Check sheet for the modelled part. Datum: model origin and axes. Units: mm. Coordinates: 2 decimals unless noted, no trailing zeros. Write each loop counter-clockwise with the first axis right and the second up, starting at its lowest first coordinate (ties: lowest second). Pieces come first, ordered by that corner, then holes. Notation, with made-up numbers: M 75.5,-32.5 L 79.5,-32.5 A24 cw 79.5,-0.5 Z; hole C 59,2 d9. An arc over 180 degrees is marked long. Answer as CSV lines item,"result".
from build123d import *
from build123d.topology import SkipClean

# Parameters (mm, degrees)
SKETCH1_R           = 39.35
BOSS_EXTRUDE1_DEPTH = 5
SKETCH2_R           = 34.4
CUT_EXTRUDE1_DEPTH  = 5
CUT_EXTRUDE2_START  = -5
CUT_EXTRUDE2_DEPTH  = 5
BOSS_EXTRUDE2_START = -5
BOSS_EXTRUDE2_DEPTH = 5
BOSS_EXTRUDE3_START = -5
BOSS_EXTRUDE3_DEPTH = 5
SKETCH11_R          = 1.5
CUT_EXTRUDE3_DEPTH  = 5
SKETCH12_R          = 1.5
CUT_EXTRUDE4_DEPTH  = 5


with BuildPart() as part:
    # Sketch1 → Boss-Extrude1 (new body)
    with BuildSketch(Plane(origin=(0, 0, 0), x_dir=(1, 0, 0), z_dir=(0, 1, 0))):
        with Locations(Location((0, 0, 0), (0, 0, 270))):
            Circle(SKETCH1_R)
    extrude(amount=BOSS_EXTRUDE1_DEPTH)

    # Sketch2 → Cut-Extrude1 (cut)
    with BuildSketch(Plane(origin=(0, 5, 0), x_dir=(1, 0, 0), z_dir=(0, 1, 0))):
        with Locations(Location((0, 0, 0), (0, 0, 270))):
            Circle(SKETCH2_R)
    extrude(amount=-CUT_EXTRUDE1_DEPTH, mode=Mode.SUBTRACT)

    # Sketch4 → Cut-Extrude2 (cut)
    with SkipClean():  # the faces are left unmerged after this step: merging them gives an invalid solid
        with BuildSketch(Plane(origin=(0, 5, 0), x_dir=(1, 0, 0), z_dir=(0, 1, 0)).offset(CUT_EXTRUDE2_START)):
            with BuildLine():
                Line((-159.77746759, -178.119268716), (-26.275583759, -29.291913528))
                Line((-26.275583759, -29.291913528), (0, 0))
                Line((0, 0), (39.349993818, 0.02205808))
                ThreePointArc((39.349993818, 0.02205808), (16.048747068, -35.928543215), (-26.275583759, -29.291913528))
                ThreePointArc((-26.275583759, -29.291913528), (16.038676365, -35.933039956), (39.35, 0))
                Line((39.35, 0), (39.35, 199.930824633))
                Line((39.35, 199.930824633), (-314.435547484, 386.277611421))
                Line((-314.435547484, 386.277611421), (-513.563015073, 8.227518071))
                Line((-513.563015073, 8.227518071), (-159.77746759, -178.119268716))
            make_face()
        extrude(amount=CUT_EXTRUDE2_DEPTH, mode=Mode.SUBTRACT)

    # Sketch9 → Boss-Extrude2 (add)
    with SkipClean():  # the faces are left unmerged after this step: merging them gives an invalid solid
        with BuildSketch(Plane(origin=(0, 5, 0), x_dir=(1, 0, 0), z_dir=(0, 1, 0)).offset(BOSS_EXTRUDE2_START)):
            with BuildLine():
                Line((-22.970268903, -25.607162016), (-26.275583759, -29.291913528))
                ThreePointArc((-26.275583759, -29.291913528), (16.048747068, -35.928543215), (39.349993818, 0.02205808))
                ThreePointArc((39.349993818, 0.02205808), (36.873606818, 2.495670303), (34.399994595, 0.019283303))
                ThreePointArc((34.399994595, 0.019283303), (14.029908491, -31.40894248), (-22.970268903, -25.607162016))
            make_face()
        extrude(amount=BOSS_EXTRUDE2_DEPTH)

    # Sketch10 → Boss-Extrude3 (add)
    with SkipClean():  # the faces are left unmerged after this step: merging them gives an invalid solid
        with BuildSketch(Plane(origin=(0, 5, 0), x_dir=(1, 0, 0), z_dir=(0, 1, 0)).offset(BOSS_EXTRUDE3_START)):
            with BuildLine():
                ThreePointArc((-26.275583759, -29.291913528), (-26.465302087, -25.796880344), (-22.970268903, -25.607162016))
                ThreePointArc((-22.970268903, -25.607162016), (14.029908491, -31.40894248), (34.399994595, 0.019283303))
                ThreePointArc((34.399994595, 0.019283303), (36.873606818, 2.495670303), (39.349993818, 0.02205808))
                ThreePointArc((39.349993818, 0.02205808), (16.048747068, -35.928543215), (-26.275583759, -29.291913528))
            make_face()
        extrude(amount=BOSS_EXTRUDE3_DEPTH)

    # Sketch11 → Cut-Extrude3 (cut)
    with SkipClean():  # the faces are left unmerged after this step: merging them gives an invalid solid
        with BuildSketch(Plane(origin=(0, 5, 0), x_dir=(1, 0, 0), z_dir=(0, 1, 0))):
            with Locations(Location((-24.622926331, -27.449537772, 0), (0, 0, 270))):
                Circle(SKETCH11_R)
        extrude(amount=-CUT_EXTRUDE3_DEPTH, mode=Mode.SUBTRACT)

    # Sketch12 → Cut-Extrude4 (cut)
    with SkipClean():  # the faces are left unmerged after this step: merging them gives an invalid solid
        with BuildSketch(Plane(origin=(0, 5, 0), x_dir=(1, 0, 0), z_dir=(0, 1, 0))):
            with Locations(Location((36.874994206, 0.020670692, 0), (0, 0, 270))):
                Circle(SKETCH12_R)
        extrude(amount=-CUT_EXTRUDE4_DEPTH, mode=Mode.SUBTRACT)


solid = part.part
1) Section check B-B, the plane z = 28. Record the boundary of the cut face in (x, y).
Answer key:
outline,"M -27.04,0 L -26.02,0 L -26.02,5 L -27.04,5 Z; M -23.23,0 L -19.98,0 L -19.98,5 L -23.23,5 Z; M 19.98,0 L 27.65,0 L 27.65,5 L 19.98,5 Z"
2) Section check D-D, the plane x = -5. Record the boundary of the cut face in (y, z), plus the area to 3 significant figures.
Answer key:
outline,"M 0,34.03 L 5,34.03 L 5,39.03 L 0,39.03 Z"
area,"25.0 mm2"
3) Thickness scan on line 1 along X through (y, z) = (1.15, 27); line 2 along X through (y, z) = (2.3, 27.5); line 3 along X through (y, z) = (1.1, 30). Record the ranges inside material, lowest first.
Answer key:
line 1,"x = -27.06 to -26.05, -23.19 to -21.32, 21.32 to 28.63"
line 2,"x = -27.1 to -26.12, -23.12 to -20.67, 20.67 to 28.15"
line 3,"x = -25.46 to -16.83, 16.83 to 25.46"
4) Section check A-A, the plane z = 33.5. Record the boundary of the cut face in (x, y).
Answer key:
outline,"M -20.64,0 L -7.82,0 L -7.82,5 L -20.64,5 Z; M 7.82,0 L 20.64,0 L 20.64,5 L 7.82,5 Z"
5) Mould release check, pull along Z, two halves, no side actions. Record for faces 1 (the face through (-26.501, 2.465, 25.838)), 2 (the face through (35.4, 2.5, -0.3)), 3 (the face through (-24.56, 2.54, 25.95)), 4 (the face through (16, 0, 31)): pulls with the +Z half, pulls with the -Z half, needs draft (parallel to the pull), parting line crosses it, or undercut.
Answer key:
face 1,"parting line crosses it"
face 2,"undercut"
face 3,"undercut"
face 4,"needs draft"
6) Depth check by flat-ended pin: P1, Ø1.5, axis at x = -0.5, y = 3, coming from the +Z side; P2, Ø1, axis at x = -6.5, y = 2, coming from the -Z side; P3, Ø3.5, axis at x = -24.62, z = 27.45, coming from the +Y side; P4, Ø1.8, axis at x = 36.87, z = -0.02, coming from the -Y side. Enter the tip coordinate at first touch or a pass-through.
Answer key:
P1,"stops at z = 39.35"
P2,"stops at z = 33.68"
P3,"stops at y = 5"
P4,"passes through"
7) Section check C-C, the plane y = 2.4. Record the boundary of the cut face in (x, z) (3 decimals).
Answer key:
outline,"M -26.276,29.292 A2.475 ccw -22.97,25.607 A34.4 cw 34.4,-0.019 A2.475 ccw 39.35,-0.022 A39.35 ccw Z; hole C -24.623,27.45 d3; hole C 36.875,-0.021 d3"
